CAD build for the part. Positions are in the model's coordinates, mm. A direction names the side the tool comes from. Round coordinates to 2 decimals unless told otherwise and drop trailing zeros. Write each loop counter-clockwise with the first axis right and the second up, starting at its lowest first coordinate (ties: lowest second). Pieces come first, ordered by that corner, then holes. Notation, with made-up numbers: (48, 74) - (90, 74) arc R34 ccw to (90, 105) - close; hole circle Ø6 at (-40, 74). An arc over 180 degrees is marked (long way). Put each result on its own line as item: value. Start each with the question number.
Item 1: Cut at A-A (x = -34.5). Give the cut face in (y, z).
Item 2: 3-axis set-ups, long thin cutter, end or side, ignore diameter. For faces 5 (the flat face through (1, 25, -52)), 6 (the flat face through (39, 0, 0)): which of +Z, -Z, +X, -X, +Y, -Y reach the whole face in a straight line?
Item 3: Cut at B-B (y = 47). Give the cut face in (x, z).
Item 4: Drill centre lines: line 1 (X direction, y = 37, z = 36); line 2 (Z direction, x = 1, y = 34). Where is each one in solid material? Low to high. Write a range as from..to.
Item 5: Cut at C-C (z = 17.5). Give the cut face in (x, y), and give its area (3 significant figures).
Item 6: Mould opens along X. For faces 1 (the flat face through (-40.81, 25, -1)), 2 (the flat face through (39, 50.8, 0)), 3 (the flat face through (-1, 25, 52)), 4 (the flat face through (-37, 25, -1)) say: released by +X, released by -X, zero draft, split by the parting line, or undercut.
Autodesk Inventor part; units mm, degrees
ref_plane "YZ Plane" through (0, 0, 0) normal (1, 0, 0) x (0, 1, 0)
ref_plane "XZ Plane" through (0, 0, 0) normal (0, 1, 0) x (-1, 0, 0)
ref_plane "XY Plane" through (0, 0, 0) normal (0, 0, 1) x (1, 0, 0)
sketch "Sketch1" plane through (0, 0, 0) normal (0, 1, 0) x (-1, 0, 0)
  line L0 (37, 52) -> (-37, 52)
  line L1 (-37, 52) -> (-37, -52)
  line L2 (-37, -52) -> (37, -52)
  line L3 (37, -52) -> (37, 52)
  line L4 (40.81, 55.81) -> (-40.81, 55.81)
  line L5 (-40.81, 55.81) -> (-40.81, -55.81)
  line L6 (-40.81, -55.81) -> (40.81, -55.81)
  line L7 (40.81, -55.81) -> (40.81, 55.81)
  point P0 (0, 0)
  point P1 (0, -52)
  point P2 (37, 0)
  dimension "d0" = 74
  dimension "d1" = 104
  dimension "d2" = 3.81
extrude "Extrusion1" add sketch "Sketch1" along normal blind 50.8
sketch "Sketch2" plane through (-40.81, 0, 55.81) normal (0, 0, 1) x (1, 0, 0)
  line L0 (3.81, 50.8) -> (77.81, 50.8)
  line L1 (40.81, 41.275) -> (40.81, 22.275)
  point P0 (40.81, 0)
  dimension "d6" = 19
properties part number "Case"
Output values:
1. outline: (0, -55.81) - (50.8, -55.81) - (50.8, -52) - (0, -52) - close; (0, 52) - (50.8, 52) - (50.8, 55.81) - (0, 55.81) - close
2. face 5: +Y, -Y
2. face 6: +Z, -Z, +X, -X, -Y
3. outline: (-40.81, -55.81) - (40.81, -55.81) - (40.81, 55.81) - (-40.81, 55.81) - close; hole (-37, -52) - (37, -52) - (37, 52) - (-37, 52) - close
4. line 1: -40.81..-37, 37..40.81
4. line 2: -55.81..-52, 52..55.81
5. outline: (-40.81, 0) - (-37, 0) - (-37, 50.8) - (-40.81, 50.8) - close; (37, 0) - (40.81, 0) - (40.81, 50.8) - (37, 50.8) - close
5. area: 387 mm2
6. face 1: released by -X
6. face 2: zero draft
6. face 3: undercut
6. face 4: undercut
